Autodesk Inventor part; units mm, degrees
ref_plane "YZ Plane" through (0, 0, 0) normal (1, 0, 0) x (0, 1, 0)
ref_plane "XZ Plane" through (0, 0, 0) normal (0, 1, 0) x (-1, 0, 0)
ref_plane "XY Plane" through (0, 0, 0) normal (0, 0, 1) x (1, 0, 0)
sketch "Sketch1" plane through (0, 0, 0) normal (1, 0, 0) x (0, 1, 0)
  circle A0 centre (0, 0) radius 3.0734
  line L0 (5.08, 5.08) -> (-5.08, 5.08)
  line L1 (-5.08, 5.08) -> (-5.08, -22.86)
  line L2 (-5.08, -22.86) -> (5.08, -22.86)
  line L3 (5.08, -22.86) -> (5.08, 5.08)
  line L4 (-5.08, -22.86) -> (12.192, -22.86)
  line L5 (12.192, -22.86) -> (12.192, -17.78)
  line L6 (12.192, -17.78) -> (-5.08, -17.78)
  line L7 (-5.08, -17.78) -> (-5.08, -22.86)
  point P0 (5.08, -17.78)
  point P1 (5.08, -22.86)
  dimension "d0" = 6.1468
  dimension "d1" = 5.08
  dimension "d2" = 5.08
  dimension "d3" = 5.08
  dimension "d4" = 22.86
  dimension "d5" = 5.08
  dimension "d6" = 7.112
extrude "Extrusion1" add sketch "Sketch1" along normal blind 5.334
sketch "Sketch2" plane through (0, 0, 0) normal (-1, 0, 0) x (0, 0, 1)
  circle A0 centre (0, 0) radius 1.5875
  circle A1 centre (0, 0) radius 3.4736
  dimension "d9" = 3.175
extrude "Extrusion2" add sketch "Sketch2" against normal blind 5.334
fillet "Fillet1" radius 5.08 3 edges at (2.667, -5.08, -22.86) (2.667, 5.08, 5.08) (2.667, -5.08, 5.08)
sketch "Sketch3" plane through (5.334, 0, 0) normal (1, 0, 0) x (0, 0, -1)
  point P0 (0, 0)
sketch "Sketch4" plane through (5.334, 0, 0) normal (1, 0, 0) x (0, 0, -1)
  circle A0 centre (0, 0) radius 5.08
  line L0 (5.08, 0) -> (23.4096, 0)
  line L1 (23.4096, 0) -> (23.4096, -6.5655)
  line L2 (23.4096, -6.5655) -> (5.08, -6.5655)
  line L3 (5.08, -6.5655) -> (5.08, 0)
  line L4 (0, -5.08) -> (17.78, -5.08)
  line L5 (0, -5.08) -> (4.9426, -5.08)
  point P0 (5.08, -5.08)
extrude "Extrusion3" cut sketch "Sketch4" against normal blind 2.54 contours L3 L4 A0 | L0 L1 L2 L3
chamfer "Chamfer1" distance 2.54 angle 45 1 edges at (5.334, 0, -13.97)
sketch "Sketch6" plane through (5.334, 0, 0) normal (1, 0, 0) x (0, 0, -1)
  circle A0 centre (0, 0) radius 3.0734
  dimension "d30" = 6.1468
extrude "Extrusion5" cut sketch "Sketch6" against normal blind 4.064 draft -4
properties part number "ServoHorn"
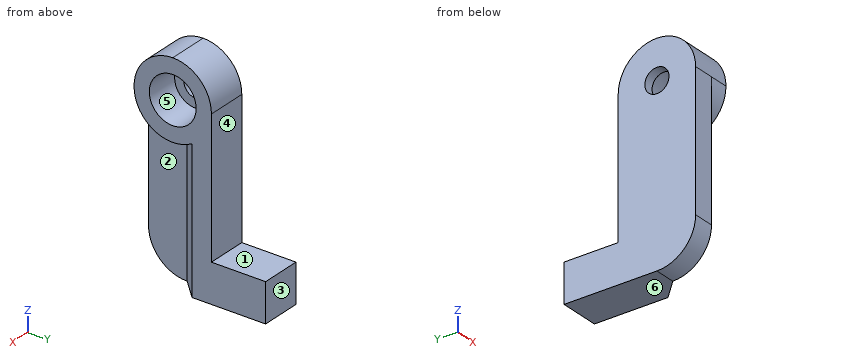
Verification items for the finished model (mm, model axes). Face numbers are marked on the shaded views. A direction names the side the tool comes from. Give positions to 0.01 mm unless a question says otherwise; leave off trailing zeros. Write each loop counter-clockwise with the first axis right and the second up, starting at its lowest first coordinate (ties: lowest second). Pieces come first, ordered by that corner, then holes. Notation, with made-up numbers: (17.25, 51.5) - (42.25, 51.5) arc R27 cw to (42.25, 68.5) - close; hole circle Ø4 at (25.5, -24). An arc over 180 degrees is marked (long way). Put each result on its own line as item: value.
Q1. Depth check by flat-ended pin: P1, Ø1.5, axis at x = 4, y = 4, coming from the +Z side; P2, Ø5.5, axis at y = -3, z = -9.5, coming from the +X side; P3, Ø1, axis at x = 4.5, y = 8, coming from the +Z side. Enter the tip coordinate at first touch or a pass-through.
Result:
P1: z = 3.9
P2: x = 2.79
P3: z = -17.78
Q2. Mould release check, pull along Z, two halves, no side actions. Record for the marked faces 4, 5 and 6: released by +Z, released by -Z, zero draft, split by the parting line, or undercut.
Result:
face 4: zero draft
face 5: undercut
face 6: released by -Z
Q3. Set-up check for the marked faces 1, 2 and 3: record each of +Z, -Z, +X, -X, +Y, -Y from which the full face is reachable in a straight line by a thin tool's end or side.
Result:
face 1: +Z, +X, -X, +Y
face 2: -Z, +X, -Y
face 3: +Z, -Z, +X, -X, +Y
Q4. Scan lines: probe 1 along Y at (x, z) = (1.05, 0); probe 2 along Z at (x, y) = (3.45, 5.75); probe 3 along X at (y, z) = (-4, -10). Record each from-to range of solid material in increasing order. Write a range as from..to.
Result:
probe 1: -5.08..-1.59, 1.59..5.08
probe 2: -22.86..-17.78
probe 3: 0..2.79
Q5. Section check C-C on y = 9. Record the cut outline in (x, z).
Result:
outline: (0, -22.86) - (5.33, -22.86) - (5.33, -17.78) - (0, -17.78) - close
